from build123d import *

# Parameters (mm, degrees)
SKETCH_W      = 25
SKETCH_H      = 18
SKETCH_R      = 2.6
PAD_DEPTH     = 2
SKETCH001_R   = 4.75
SKETCH001_R_2 = 2.6
PAD001_DEPTH  = 1


with BuildPart() as part:
    # Sketch → Pad (new body)
    with BuildSketch(Plane.XY):
        Rectangle(SKETCH_W, SKETCH_H)
        with Locations((-7.5, 0)):
            Circle(SKETCH_R, mode=Mode.SUBTRACT)
        with Locations((7.5, 0)):
            Circle(SKETCH_R, mode=Mode.SUBTRACT)
    extrude(amount=PAD_DEPTH)

    # Sketch001 (on Face8 of Pad) → Pad001 (join)
    with BuildSketch(Plane.XY.offset(2)):
        with Locations((-7.5, 0)):
            Circle(SKETCH001_R)
        with Locations((-7.5, 0)):
            Circle(SKETCH001_R_2, mode=Mode.SUBTRACT)
        with Locations((7.5, 0)):
            Circle(SKETCH001_R)
        with Locations((7.5, 0)):
            Circle(SKETCH001_R_2, mode=Mode.SUBTRACT)
    extrude(amount=PAD001_DEPTH)


solid = part.part
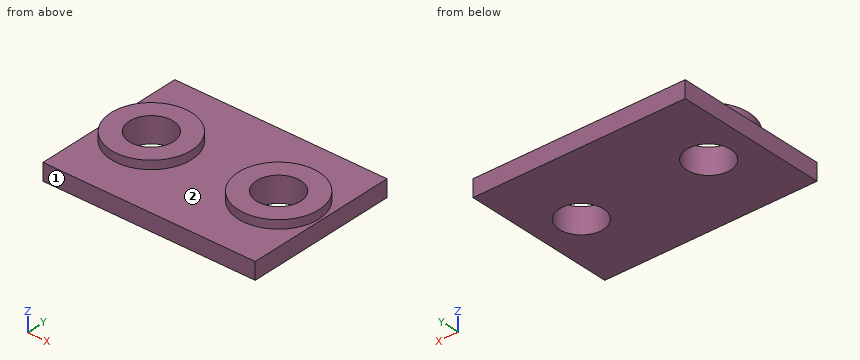
The listing builds one solid part. Answer for the finished solid, in the listing's coordinates (mm). Face numbers are marked on the shaded views. Coordinates: 2 decimals unless noted, no trailing zeros. Loops run counter-clockwise (first coordinate to the right, second up) from the corner with the lowest first, then second, coordinate; pieces in that order, holes last.
1) Find section A-A on x = -7.5. Write down the section's boundary in (y, z), then the cut area to 3 significant figures.
2) Find the intervals of material crossed by L1, parallel to X at y = 0.25, z = 1.1; L2, parallel to Z at x = -10.25, y = 7.5; L3, parallel to X at y = 2, z = 1.1, in increasing order.
3) Find section B-B on y = 0. Write down the section's boundary in (x, z).
4) Flat-ended cylindrical pins translate along their axes: pin 1 Ø1 at (x, y) = (0, -3) entering from +Z; pin 2 Ø8.5 at (x, y) = (7.5, 0) entering from -Z. Find the tip coordinate at first contact, or state that the pin passes through.
5) Find section D-D on x = -3. Write down the section's boundary in (y, z), then the cut area to 3 significant figures.
6) Find section C-C on z = 1.75. Write down the section's boundary in (x, y), then the cut area to 3 significant figures.
7) Determine the mould class of the marked faces 1 and 2 for opening direction X: pulls with the +X half, pulls with the -X half, needs draft (parallel to the pull), parting line crosses it, or undercut.
Values:
1. outline: (-9, 0) - (-2.6, 0) - (-2.6, 3) - (-4.75, 3) - (-4.75, 2) - (-9, 2) - close; (2.6, 0) - (9, 0) - (9, 2) - (4.75, 2) - (4.75, 3) - (2.6, 3) - close
1. area: 29.9 mm2
2. L1: x = -12.5 to -10.09, -4.91 to 4.91, 10.09 to 12.5
2. L2: z = 0 to 2
2. L3: x = -12.5 to -9.16, -5.84 to 5.84, 9.16 to 12.5
3. outline: (-12.5, 0) - (-10.1, 0) - (-10.1, 3) - (-12.25, 3) - (-12.25, 2) - (-12.5, 2) - close; (-4.9, 0) - (4.9, 0) - (4.9, 3) - (2.75, 3) - (2.75, 2) - (-2.75, 2) - (-2.75, 3) - (-4.9, 3) - close; (10.1, 0) - (12.5, 0) - (12.5, 2) - (12.25, 2) - (12.25, 3) - (10.1, 3) - close
4. pin 1: stops at z = 2
4. pin 2: stops at z = 0
5. outline: (-9, 0) - (9, 0) - (9, 2) - (1.52, 2) - (1.52, 3) - (-1.52, 3) - (-1.52, 2) - (-9, 2) - close
5. area: 39.0 mm2
6. outline: (-12.5, -9) - (12.5, -9) - (12.5, 9) - (-12.5, 9) - close; hole circle Ø5.2 at (-7.5, 0); hole circle Ø5.2 at (7.5, 0)
6. area: 408 mm2
7. face 1: needs draft
7. face 2: undercut
